Could you check a few things on this model? Use its own coordinates, in mm. Face numbers are marked on the shaded views. A direction names the side the tool comes from. Give positions to 0.01 mm unless a question says otherwise; leave off trailing zeros. Write each loop counter-clockwise with the first axis right and the second up, starting at its lowest first coordinate (ties: lowest second). Pieces come first, ordered by that corner, then holes. Notation, with made-up numbers: (44.5, 51.25) - (72.5, 51.25) arc R35 cw to (72.5, 83.25) - close; hole circle Ø7 at (71.25, -32.5). An arc over 180 degrees is marked (long way). Answer as CSV lines item,"result". Start each with the question number.
Q1. Imagine slicing it at A-A on x = 4. List the corners of the cut face in (y, z) for me.
Q2. On a 3-axis mill with a long thin cutter (end or side, diameter ignored), from which of +Z, -Z, +X, -X, +Y, -Y can I reach the whole of each face in a straight line? I mean the marked faces 1, 2 and 3. Say none if no direction works.
Q3. Will these pins go through, and if not, where does the flat tip stop? pin 1 Ø1.5 at (x, y) = (17.5, -1) entering from +Z; pin 2 Ø2 at (x, z) = (60.5, 5.5) entering from +Y.
Q4. Imagine slicing it at B-B on y = 21.4. List the corners of the cut face in (x, z) for me.
Q5. Imagine slicing it at D-D on z = 4. State how many separate pieces and enclosed holes the cut face has, and give its area (3 significant figures).
Q6. Imagine slicing it at C-C on x = 12. List the corners of the cut face in (y, z) for me, and give its area (3 significant figures).
Q7. If I drill on line 1 along Z through (x, y) = (70.5, 27.5); line 2 along X through (y, z) = (23, 5.75); line 3 along Y through (x, z) = (44, 5.25), over which ranges is the centre line in solid material (lowest first)?
```python
from build123d import *

# Parameters (mm, degrees)
SKETCH1_R           = 2.5
BOSS_EXTRUDE1_DEPTH = 1.5
BOSS_EXTRUDE2_START = 7.5
SKETCH1_13_R        = 2.5
BOSS_EXTRUDE2_DEPTH = 7.5
BOSS_EXTRUDE3_START = 9
SKETCH1_14_R        = 2.5
BOSS_EXTRUDE3_DEPTH = 1.5


with BuildPart() as part:
    # Sketch1 → Boss-Extrude1 (new body)
    # profile 1 of 9: a face of its own
    with BuildSketch(Plane.XY):
        Polygon((0, 87.5), (0, 82.275), (20, 86), (45, 51), (75, 51), (75, 52.5), (45, 52.5), (20, 87.5), align=None)
    # profile 2 of 9: a face of its own
    with BuildSketch(Plane.XY):
        Polygon((0, 82.275), (0, 72.275), (20, 68.55), (45, 32.875), (75, 32.875), (75, 51), (45, 51), (20, 86), align=None)
    # profile 3 of 9: a face of its own
    with BuildSketch(Plane.XY):
        Polygon((0, 72.275), (0, 59.925), (20, 63.65), (45, 31.375), (75, 31.375), (75, 32.875), (45, 32.875), (20, 68.55), align=None)
    # profile 4 of 9: a face of its own
    with BuildSketch(Plane.XY):
        Polygon((0, 59.925), (0, 49.925), (20, 46.2), (45, 13.25), (75, 13.25), (75, 31.375), (45, 31.375), (20, 63.65), align=None)
    # profile 5 of 9: a face of its own
    with BuildSketch(Plane.XY):
        Polygon((0, 49.925), (0, 37.575), (20, 41.3), (45, 11.75), (75, 11.75), (75, 13.25), (45, 13.25), (20, 46.2), align=None)
    # profile 6 of 9: a face of its own
    with BuildSketch(Plane.XY):
        Polygon((0, 37.575), (0, 27.575), (20, 23.85), (45, -6.375), (75, -6.375), (75, 11.75), (45, 11.75), (20, 41.3), align=None)
    # profile 7 of 9: a face of its own
    with BuildSketch(Plane.XY):
        Polygon((0, 27.575), (0, 15.225), (20, 18.95), (45, -7.875), (75, -7.875), (75, -6.375), (45, -6.375), (20, 23.85), align=None)
        with Locations((4, 21.4)):
            Circle(SKETCH1_R, mode=Mode.SUBTRACT)
    # profile 8 of 9: a face of its own
    with BuildSketch(Plane.XY):
        Polygon((0, 15.225), (0, 5.225), (20, 1.5), (45, -26), (75, -26), (75, -7.875), (45, -7.875), (20, 18.95), align=None)
    # profile 9 of 9: a face of its own
    with BuildSketch(Plane.XY):
        Polygon((0, 5.225), (0, 0), (20, 0), (45, -27.5), (75, -27.5), (75, -26), (45, -26), (20, 1.5), align=None)
    extrude(amount=-BOSS_EXTRUDE1_DEPTH)

    # Sketch1_13 → Boss-Extrude2 (add)
    # profile 1 of 5: a face of its own
    with BuildSketch(Plane.XY.offset(BOSS_EXTRUDE2_START)):
        Polygon((0, 87.5), (0, 82.275), (20, 86), (45, 51), (75, 51), (75, 52.5), (45, 52.5), (20, 87.5), align=None)
    # profile 2 of 5: a face of its own
    with BuildSketch(Plane.XY.offset(BOSS_EXTRUDE2_START)):
        Polygon((0, 72.275), (0, 59.925), (20, 63.65), (45, 31.375), (75, 31.375), (75, 32.875), (45, 32.875), (20, 68.55), align=None)
    # profile 3 of 5: a face of its own
    with BuildSketch(Plane.XY.offset(BOSS_EXTRUDE2_START)):
        Polygon((0, 49.925), (0, 37.575), (20, 41.3), (45, 11.75), (75, 11.75), (75, 13.25), (45, 13.25), (20, 46.2), align=None)
    # profile 4 of 5: a face of its own
    with BuildSketch(Plane.XY.offset(BOSS_EXTRUDE2_START)):
        Polygon((0, 27.575), (0, 15.225), (20, 18.95), (45, -7.875), (75, -7.875), (75, -6.375), (45, -6.375), (20, 23.85), align=None)
        with Locations((4, 21.4)):
            Circle(SKETCH1_13_R, mode=Mode.SUBTRACT)
    # profile 5 of 5: a face of its own
    with BuildSketch(Plane.XY.offset(BOSS_EXTRUDE2_START)):
        Polygon((0, 5.225), (0, 0), (20, 0), (45, -27.5), (75, -27.5), (75, -26), (45, -26), (20, 1.5), align=None)
    extrude(amount=-BOSS_EXTRUDE2_DEPTH)

    # Sketch1_14 → Boss-Extrude3 (add)
    # profile 1 of 9: a face of its own
    with BuildSketch(Plane.XY.offset(BOSS_EXTRUDE3_START)):
        Polygon((0, 5.225), (0, 0), (20, 0), (45, -27.5), (75, -27.5), (75, -26), (45, -26), (20, 1.5), align=None)
    # profile 2 of 9: a face of its own
    with BuildSketch(Plane.XY.offset(BOSS_EXTRUDE3_START)):
        Polygon((0, 15.225), (0, 5.225), (20, 1.5), (45, -26), (75, -26), (75, -7.875), (45, -7.875), (20, 18.95), align=None)
    # profile 3 of 9: a face of its own
    with BuildSketch(Plane.XY.offset(BOSS_EXTRUDE3_START)):
        Polygon((0, 27.575), (0, 15.225), (20, 18.95), (45, -7.875), (75, -7.875), (75, -6.375), (45, -6.375), (20, 23.85), align=None)
        with Locations((4, 21.4)):
            Circle(SKETCH1_14_R, mode=Mode.SUBTRACT)
    # profile 4 of 9: a face of its own
    with BuildSketch(Plane.XY.offset(BOSS_EXTRUDE3_START)):
        Polygon((0, 37.575), (0, 27.575), (20, 23.85), (45, -6.375), (75, -6.375), (75, 11.75), (45, 11.75), (20, 41.3), align=None)
    # profile 5 of 9: a face of its own
    with BuildSketch(Plane.XY.offset(BOSS_EXTRUDE3_START)):
        Polygon((0, 49.925), (0, 37.575), (20, 41.3), (45, 11.75), (75, 11.75), (75, 13.25), (45, 13.25), (20, 46.2), align=None)
    # profile 6 of 9: a face of its own
    with BuildSketch(Plane.XY.offset(BOSS_EXTRUDE3_START)):
        Polygon((0, 59.925), (0, 49.925), (20, 46.2), (45, 13.25), (75, 13.25), (75, 31.375), (45, 31.375), (20, 63.65), align=None)
    # profile 7 of 9: a face of its own
    with BuildSketch(Plane.XY.offset(BOSS_EXTRUDE3_START)):
        Polygon((0, 72.275), (0, 59.925), (20, 63.65), (45, 31.375), (75, 31.375), (75, 32.875), (45, 32.875), (20, 68.55), align=None)
    # profile 8 of 9: a face of its own
    with BuildSketch(Plane.XY.offset(BOSS_EXTRUDE3_START)):
        Polygon((0, 82.275), (0, 72.275), (20, 68.55), (45, 32.875), (75, 32.875), (75, 51), (45, 51), (20, 86), align=None)
    # profile 9 of 9: a face of its own
    with BuildSketch(Plane.XY.offset(BOSS_EXTRUDE3_START)):
        Polygon((0, 87.5), (0, 82.275), (20, 86), (45, 51), (75, 51), (75, 52.5), (45, 52.5), (20, 87.5), align=None)
    extrude(amount=-BOSS_EXTRUDE3_DEPTH)


solid = part.part
```
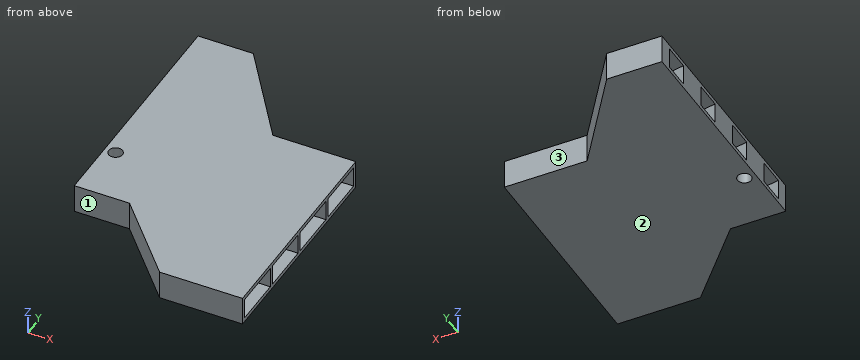
Conclusion:
1,outline,"(0, -1.5) - (18.9, -1.5) - (18.9, 9) - (0, 9) - close; (23.9, -1.5) - (87.5, -1.5) - (87.5, 9) - (23.9, 9) - close; hole (4.48, 0) - (15.97, 0) - (15.97, 7.5) - (4.48, 7.5) - close; hole (26.83, 0) - (38.32, 0) - (38.32, 7.5) - (26.83, 7.5) - close; hole (49.18, 0) - (60.67, 0) - (60.67, 7.5) - (49.18, 7.5) - close; hole (71.53, 0) - (83.02, 0) - (83.02, 7.5) - (71.53, 7.5) - close"
2,face 1,"+Z, -Z, -X, -Y"
2,face 2,"-Z, +X, -X, +Y, -Y"
2,face 3,"+Z, -Z, +X, +Y"
3,pin 1,"through"
3,pin 2,"y = 52.5"
4,outline,"(0, -1.5) - (1.5, -1.5) - (1.5, 9) - (0, 9) - close; (6.5, -1.5) - (75, -1.5) - (75, 0) - (38.82, 0) - (38.82, 7.5) - (75, 7.5) - (75, 9) - (6.5, 9) - close; hole (22.03, 0) - (36.84, 0) - (36.84, 7.5) - (22.03, 7.5) - close"
5,separate pieces,"5"
5,enclosed holes,"1"
5,area,"1,170 mm^2"
6,outline,"(0, -1.5) - (87.5, -1.5) - (87.5, 9) - (0, 9) - close; hole (2.99, 0) - (17.46, 0) - (17.46, 7.5) - (2.99, 7.5) - close; hole (25.34, 0) - (39.81, 0) - (39.81, 7.5) - (25.34, 7.5) - close; hole (47.69, 0) - (62.16, 0) - (62.16, 7.5) - (47.69, 7.5) - close; hole (70.04, 0) - (84.51, 0) - (84.51, 7.5) - (70.04, 7.5) - close"
6,area,"485 mm^2"
7,line 1,"-1.5 to 0, 7.5 to 9"
7,line 2,"0 to 2.08, 5.92 to 20.7, 35.48 to 37.6"
7,line 3,"-26.4 to -24.9, -6.8 to -5.17, 12.93 to 14.57, 32.67 to 34.3, 52.4 to 53.9"
